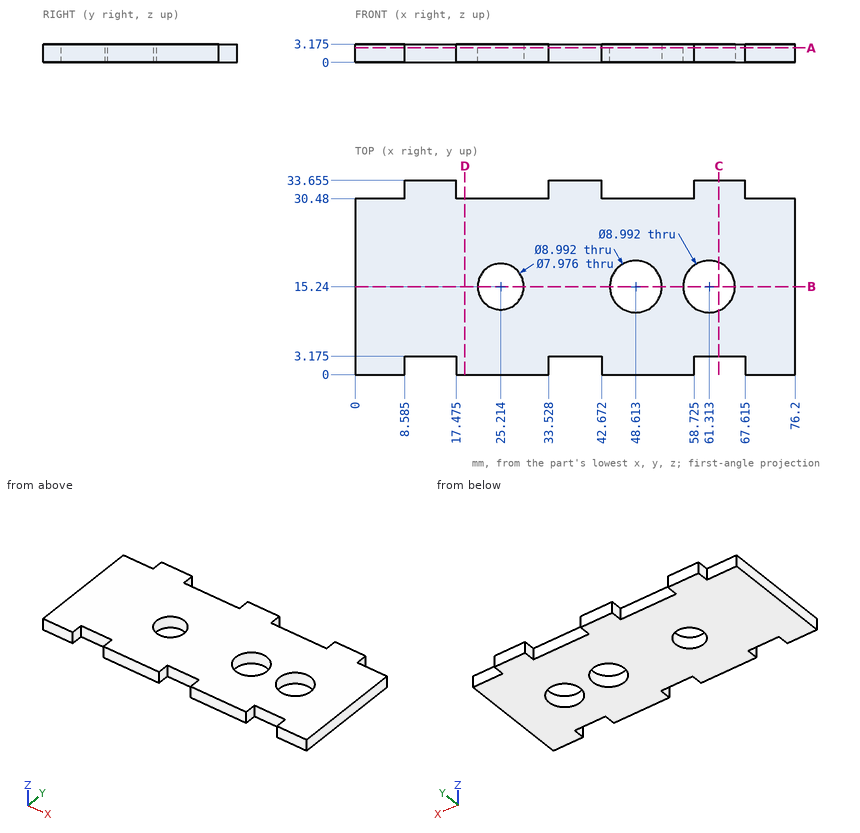
Here's the drawing with two shaded views (mm, measured from the low corner). I have some questions. Give positions to 0.01 mm unless a question says otherwise; leave off trailing zeros. Write each loop counter-clockwise with the first axis right and the second up, starting at its lowest first coordinate (ties: lowest second). Pieces come first, ordered by that corner, then holes. Notation, with made-up numbers: (-29.75, 78.5) -> (14.25, 78.5) arc R23 cw to (14.25, 115.5) -> close; hole circle Ø10 at (80, 0.25). An arc over 180 degrees is marked (long way). Answer as a JSON object with one key per item and string values. Group by question number.
Item 1: Suppose I cut it at C-C (x = 63). Please give me the cut outline in (y, z) (1 decimal).
Item 2: Suppose I cut it at B-B (y = 15.24). Please give me the cut outline in (x, z) (1 decimal).
Item 3: Suppose I cut it at D-D (x = 19). Please give me the cut outline in (y, z) (1 decimal).
Item 4: Please list where these lines run through material, in increasing order: line 1 (X direction, y = 2, z = 1.1) (1 decimal); line 2 (Y direction, x = 25.5, z = 2.25); line 3 (Y direction, x = 30.5, z = 0.15). Write a range as [from, to].
Item 5: Suppose I cut it at A-A (z = 2.5). State how many separate pieces and enclosed holes the cut face has, plus the area to 3 significant figures.
Item 6: I'm going to push flat-ended pins straight in: P1, Ø1, axis at y = 32, z = 1, coming from the -X side (1 decimal); P2, Ø1, axis at x = 47, z = 0.5, coming from the +Y side; P3, Ø1.5, axis at x = 36, z = 0.5, coming from the -Y side (3 decimals). Where does each tip first touch, or does it pass through?
Findings:
{
 "1": {"outline": "(3.2, 0) -> (11.1, 0) -> (11.1, 3.2) -> (3.2, 3.2) -> close; (19.4, 0) -> (33.7, 0) -> (33.7, 3.2) -> (19.4, 3.2) -> close"},
 "2": {"outline": "(0, 0) -> (21.2, 0) -> (21.2, 3.2) -> (0, 3.2) -> close; (29.2, 0) -> (44.1, 0) -> (44.1, 3.2) -> (29.2, 3.2) -> close; (53.1, 0) -> (56.8, 0) -> (56.8, 3.2) -> (53.1, 3.2) -> close; (65.8, 0) -> (76.2, 0) -> (76.2, 3.2) -> (65.8, 3.2) -> close"},
 "3": {"outline": "(0, 0) -> (30.5, 0) -> (30.5, 3.2) -> (0, 3.2) -> close"},
 "4": {"line 1": "x = [0, 8.6], [17.5, 33.5], [42.7, 58.7], [67.6, 76.2]", "line 2": "y = [0, 11.26], [19.22, 30.48]", "line 3": "y = [0, 30.48]"},
 "5": {"separate pieces": "1", "enclosed holes": "3", "area": "2,150 mm²"},
 "6": {"P1": "stops at x = 8.6", "P2": "stops at y = 30.48", "P3": "stops at y = 3.175"}
}
